Source: three-view drawing plus pictorial views. Frame: mm from the lowest corner of the part. Give positions to 0.01 mm unless a question says otherwise; leave off trailing zeros. Order: outer loops, then holes, each group sorted by start corner. A loop starts at its lowest first (then second) coordinate and runs counter-clockwise, first axis right, second up. Notation, with made-up numbers: (54, 26) - (110, 26) arc R20 ccw to (110, 35) - close; hole circle Ø1 at (78, 62.25). An arc over 180 degrees is marked (long way). Use CSV: the item, a comma, the result in double quotes.
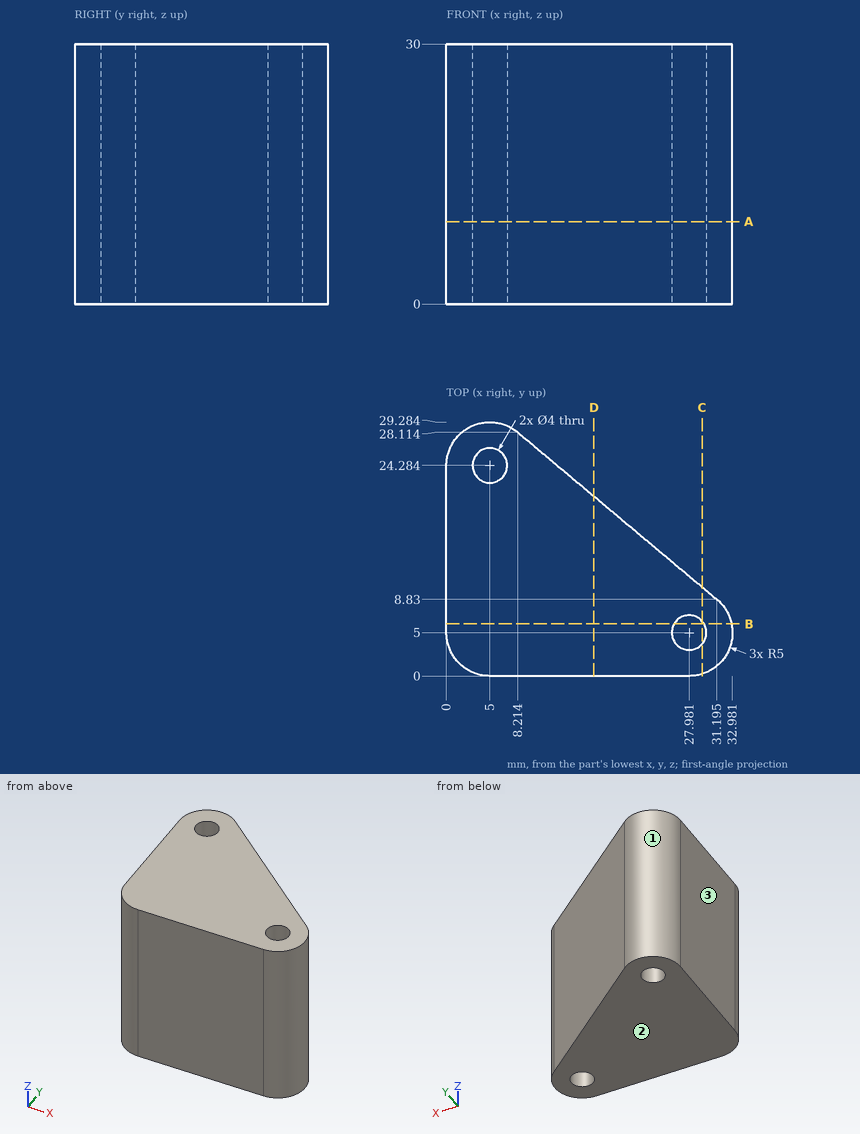
Item 1: Section B-B on y = 6. Return the cut outline in (x, z).
Filled in:
outline,"(0, 0) - (26.25, 0) - (26.25, 30) - (0, 30) - close; (29.71, 0) - (32.88, 0) - (32.88, 30) - (29.71, 30) - close"
Item 2: Section D-D on x = 17. Return the cut outline in (y, z), then the cut area to 3 significant figures.
Filled in:
outline,"(0, 0) - (20.74, 0) - (20.74, 30) - (0, 30) - close"
area,"622 mm2"
Item 3: Mould query, pull axis X, two halves, no side actions, for the marked faces 1, 2 and 3. Classes: released by +X, released by -X, zero draft, split by the parting line, or undercut.
Filled in:
face 1,"split by the parting line"
face 2,"zero draft"
face 3,"released by -X"
Item 4: Section C-C on x = 29.5. Return the cut outline in (y, z).
Filled in:
outline,"(0.24, 0) - (3.7, 0) - (3.7, 30) - (0.24, 30) - close; (6.3, 0) - (10.25, 0) - (10.25, 30) - (6.3, 30) - close"
Item 5: First-contact query: pin 1 (5 mm diameter, centred on x = 20.5, z = 6, fed in from +Y); pin 2 (8 mm diameter, centred on x = 22.5, z = 3, fed in from -Y); pin 3 (1 mm diameter, centred on x = 16, z = 23, fed in from +Y); pin 4 (2 mm diameter, centred on y = 19, z = 3.5, fed in from +X). Flat tips, straight axial feed; report the tip coordinate or a pass-through.
Filled in:
pin 1,"stops at y = 19.9"
pin 2,"stops at y = 0"
pin 3,"stops at y = 22"
pin 4,"stops at x = 20.27"
Item 6: Material intervals for line 1 (Y direction, x = 4.5, z = 2) (1 decimal); line 2 (Y direction, x = 27, z = 9.75); line 3 (Y direction, x = 31.5, z = 2.75), sorted ascending. Write a range as from..to.
Filled in:
line 1,"y = 0..22.3, 26.2..29.3"
line 2,"y = 0..3.26, 6.74..12.35"
line 3,"y = 1.45..8.55"
Item 7: Section A-A on z = 9.5. Return the cut outline in (x, y) (1 decimal).
Filled in:
outline,"(0, 5) arc R5 ccw to (5, 0) - (28, 0) arc R5 ccw to (31.2, 8.8) - (8.2, 28.1) arc R5 ccw to (0, 24.3) - close; hole circle Ø4 at (5, 24.3); hole circle Ø4 at (28, 5)"
